from build123d import *

# Parameters (mm, degrees)
F0_R     = 12.5
F1_DEPTH = 317.5
F4_D     = 8.8
F5_SIZE  = 1


with BuildPart() as f1:
    # F0 (on Right) → F1 (new body, symmetric)
    with BuildSketch(Plane.YZ):
        Circle(F0_R)
    extrude(amount=F1_DEPTH, both=True)

    # F4 (through all)
    with Locations(Plane.XZ.offset(25)):
        with Locations((-224, 0), (224, 0)):
            Hole(F4_D / 2)

    # F5
    f5_edges = [f1.edges().sort_by_distance(p)[0] for p in [
        (317.5, -12.5, 0),
        (-317.5, -12.5, 0),
    ]]
    chamfer(f5_edges, length=F5_SIZE)


solid = f1.part
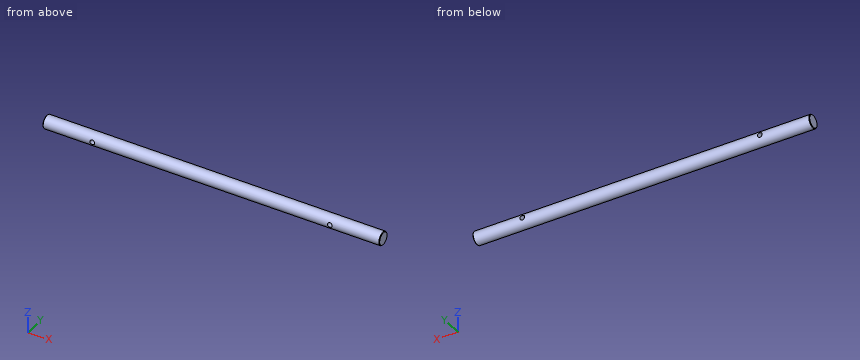
Read the model definition and answer for the solid it produces. Units are mm, in the model's axes. Round coordinates to 2 decimals unless told otherwise and drop trailing zeros. Write each loop counter-clockwise with the first axis right and the second up, starting at its lowest first coordinate (ties: lowest second). Pieces come first, ordered by that corner, then holes.
1. Straight lines are drawn through the part: L1, parallel to X at y = -5.25, z = 0; L2, parallel to X at y = -1.5, z = -4; L3, parallel to Z at x = 224, y = -1.25. For each, find the intervals that lie inside material, in ascending order.
2. The part is cut by section C-C, the plane x = -144. Determine the outline of the cut face in (y, z), then the cut area to 3 significant figures.
3. The part is cut by section A-A, the plane z = 0. Determine the outline of the cut face in (x, y), then the cut area to 3 significant figures.
4. Given pin 1 Ø1.5 at (x, y) = (-69.5, -6) entering from +Z; pin 2 Ø8 at (x, y) = (-179.5, -7) entering from +Z; pin 3 Ø7 at (x, z) = (224, 0) entering from +Y; pin 4 Ø2 at (x, y) = (11.5, 2) entering from +Z, each flat-ended and moving along its own axis, determine where each tip first touches the part or whether it passes through.
5. The part is cut by section B-B, the plane y = -7.25. State how many separate pieces and enclosed holes the cut face has, then the cut area to 3 significant figures.
Values:
1. L1: x = -317.5 to -228.4, -219.6 to 219.6, 228.4 to 317.5
1. L2: x = -317.5 to -225.83, -222.17 to 222.17, 225.83 to 317.5
1. L3: z = -12.44 to -4.4, 4.4 to 12.44
2. outline: circle Ø25 at (0, 0)
2. area: 491 mm2
3. outline: (-317.5, -11.5) - (-316.5, -12.5) - (-228.4, -12.5) - (-228.4, 12.5) - (-316.5, 12.5) - (-317.5, 11.5) - close; (-219.6, -12.5) - (219.6, -12.5) - (219.6, 12.5) - (-219.6, 12.5) - close; (228.4, -12.5) - (316.5, -12.5) - (317.5, -11.5) - (317.5, 11.5) - (316.5, 12.5) - (228.4, 12.5) - close
3. area: 15,400 mm2
4. pin 1: stops at z = 11.34
4. pin 2: stops at z = 12.13
4. pin 3: passes through
4. pin 4: stops at z = 12.46
5. separate pieces: 1
5. enclosed holes: 2
5. area: 12,800 mm2
